from build123d import *

# Parameters (mm, degrees)
F0_R     = 50
F0_R_2   = 45
F1_DEPTH = 1
F2_R     = 45.75
F3_DEPTH = 14
F5_R     = 45
F6_DEPTH = 17
F7_R     = 4.99999


# Not quite as in the source:
# - a fillet or chamfer that OpenCascade refuses, or shapes differently, is made with other operations: its cross-section is extruded or revolved along the edge and cut away or added
# - a fillet or chamfer is up to 0.001 mm smaller than in the source, because OpenCascade refuses the exact size


with BuildPart() as f1:
    # F0 (on Front) → F1 (new body)
    with BuildSketch(Plane.XZ):
        Circle(F0_R)
        Circle(F0_R_2, mode=Mode.SUBTRACT)
    extrude(amount=F1_DEPTH)

    # F2 (on Front) → F3 (join)
    with BuildSketch(Plane.XZ):
        Circle(F2_R)
    extrude(amount=F3_DEPTH)

    # F4: fillet of radius 5 on 1 edges, made by hand

    # F4_s1 → F4_t2 (revolve)
    with BuildSketch(Plane.XY):
        with BuildLine():
            ThreePointArc((49.9999399343, -0.9996045356), (46.9582217487, -2.6840834341), (45.7496, -5.9442601394))
            Line((45.7496, -5.9442601394), (45.2494634315, -5.9442601394))
            ThreePointArc((45.2494634315, -5.9442601394), (45.2498634315, -3.4721300697), (45.2498634315, -1))
            Line((45.2498634315, -1), (45.75, -0.4998634315))
            ThreePointArc((45.75, -0.4998634315), (47.8749699672, -0.4998634315), (49.9248373592, -0.5051389752))
            Line((49.9248373592, -0.5051389752), (49.9999399343, -0.9996045356))
        make_face()
    revolve(axis=Axis((0, -1, 0), (0, 1, 0)))

    # F5 (on face) → F6 (cut)
    with BuildSketch(Plane.XZ.offset(14)):
        Circle(F5_R)
    extrude(amount=-F6_DEPTH, mode=Mode.SUBTRACT)

    # F7 (radius 5 in the source; OpenCascade refuses exactly that, so slightly less here)
    f7_edges = [f1.edges().sort_by_distance(p)[0] for p in [
        (-45, 0, 0),
    ]]
    fillet(f7_edges, radius=F7_R)


solid = f1.part
The listing builds one solid part. Answer for the finished solid, in the listing's coordinates (mm). Give positions to 0.01 mm unless a question says otherwise; leave off trailing zeros. Write each loop counter-clockwise with the first axis right and the second up, starting at its lowest first coordinate (ties: lowest second). Pieces come first, ordered by that corner, then holes.
1) Given P1, Ø4, axis at y = -6, z = -37, coming from the -X side; P2, Ø1.5, axis at y = -2.5, z = -14.5, coming from the +X side; P3, Ø1.5, axis at y = -11.5, z = -5, coming from the +X side, each flat-ended and moving along its own axis, determine where each tip first touches the part or whether it passes through.
2) Find the intervals of material crossed by L1, parallel to Z at x = 0, y = -7.5; L2, parallel to Z at x = 30.5, y = -7; L3, parallel to X at y = -10.75, z = -15, in increasing order.
3) For a pull along Z with two mould halves and no side action, classify faces 1 (the face through (47.69, -0.49, 15.02)), 2 (the face through (34, -14, -30)), 3 (the face through (20.765, -9.563, -39.923)) as pulls with the +Z half, pulls with the -Z half, needs draft (parallel to the pull), parting line crosses it, or undercut.
4) Section C-C (y = -8.25) is taken. Write down the section's boundary in (x, z).
Response:
1. P1: stops at x = -29.46
1. P2: stops at x = 45.81
1. P3: stops at x = 45.55
2. L1: z = -45.75 to -45, 45 to 45.75
2. L2: z = -34.1 to -33.09, 33.09 to 34.1
2. L3: x = -43.22 to -42.43, 42.43 to 43.22
3. face 1: parting line crosses it
3. face 2: needs draft
3. face 3: undercut
4. outline: circle Ø91.5 at (0, 0); hole circle Ø90 at (0, 0)
